Design review of the part built by this model. Coordinates are the model's own, in mm. Face numbers are marked on the shaded views. A direction names the side the tool comes from. Give positions to 0.01 mm unless a question says otherwise; leave off trailing zeros. Loops run counter-clockwise (first coordinate to the right, second up) from the corner with the lowest first, then second, coordinate; pieces in that order, holes last.
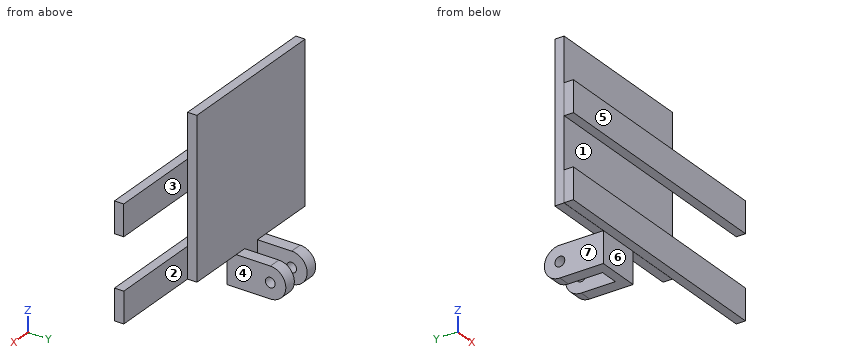
from build123d import *

# Parameters (mm, degrees)
SKETCH1_W           = 6
SKETCH1_H           = 10.023203152
BOSS_EXTRUDE1_DEPTH = 3
SKETCH1_3_W         = 4
SKETCH1_3_H         = 10.023203152
BOSS_EXTRUDE2_DEPTH = 19.05
SKETCH2_R           = 1.5875
CUT_EXTRUDE1_DEPTH  = 19.05
SKETCH3_W           = 80.796379589
SKETCH3_H           = 10
BOSS_EXTRUDE3_DEPTH = 3


with BuildPart() as part:
    # Sketch1 → Boss-Extrude1 (new body)
    with BuildSketch(Plane(origin=(0, 0, 0), x_dir=(1, 0, 0), z_dir=(0, 1, 0))):
        Polygon((0, 50.8), (0, 0), (50.8, 0), (50.8, 50.8), (32.4, 50.8), (28.4, 50.8), (22.4, 50.8), (18.4, 50.8), align=None)
        with Locations((25.4, 55.811601576)):
            Rectangle(SKETCH1_W, SKETCH1_H)
    extrude(amount=BOSS_EXTRUDE1_DEPTH)

    # Sketch1_3 → Boss-Extrude2 (add)
    with BuildSketch(Plane(origin=(0, 0, 0), x_dir=(1, 0, 0), z_dir=(0, 1, 0))):
        with Locations((30.4, 55.811601576)):
            Rectangle(SKETCH1_3_W, SKETCH1_3_H)
        with Locations((20.4, 55.811601576)):
            Rectangle(SKETCH1_3_W, SKETCH1_3_H)
    extrude(amount=BOSS_EXTRUDE2_DEPTH)

    # Sketch2 → Cut-Extrude1 (cut)
    with BuildSketch(Plane(origin=(32.4, 0, 0), x_dir=(0, 0, -1), z_dir=(1, 0, 0))):
        with Locations((55.811601576, 14.038398424)):
            Circle(SKETCH2_R)
        with BuildLine():
            Line((50.8, 14.038398424), (49.911458456, 20.395059664))
            Line((49.911458456, 20.395059664), (64.501767063, 21.247740037))
            Line((64.501767063, 21.247740037), (60.823203152, 14.038398424))
            ThreePointArc((60.823203152, 14.038398424), (55.811601576, 19.05), (50.8, 14.038398424))
        make_face()
    extrude(amount=-CUT_EXTRUDE1_DEPTH, mode=Mode.SUBTRACT)

    # Sketch3 → Boss-Extrude3 (add)
    with BuildSketch(Plane.XZ):
        Polygon((30.017240132, -14.222777316), (0.017240132, -14.222777316), (0.017240132, -24.222777316), (80.817240132, -24.222777316), (80.817240132, -14.222777316), align=None)
        with Locations((40.354723884, -45.757439596)):
            Rectangle(SKETCH3_W, SKETCH3_H)
    extrude(amount=BOSS_EXTRUDE3_DEPTH)


solid = part.part
Q1. Take a section at B-B (x = 31). Give the boundary of the cut face in (y, z) (1 decimal).
Results:
outline: (-3, -50.8) - (0, -50.8) - (0, -60.8) - (14, -60.8) arc R5 ccw to (14, -50.8) - (3, -50.8) - (3, 0) - (0, 0) - (0, -14.2) - (-3, -14.2) - (-3, -24.2) - (0, -24.2) - (0, -40.8) - (-3, -40.8) - close; hole circle Ø3.2 at (14, -55.8)
Q2. Draft analysis for pull direction Z (two halves, no side actions). For the marked faces 1 and 2, state which applies: pulls with the +Z half, pulls with the -Z half, needs draft (parallel to the pull), parting line crosses it, or undercut.
Results:
face 1: undercut
face 2: needs draft
Q3. Take a section at D-D (y = 7.75). Give the boundary of the cut face in (x, z), plus the area to 3 significant figures.
Results:
outline: (18.4, -60.82) - (22.4, -60.82) - (22.4, -50.8) - (18.4, -50.8) - close; (28.4, -60.82) - (32.4, -60.82) - (32.4, -50.8) - (28.4, -50.8) - close
area: 80.2 mm2
Q4. Take a section at A-A (x = 73). Give the boundary of the cut face in (y, z).
Results:
outline: (-3, -50.76) - (0, -50.76) - (0, -40.76) - (-3, -40.76) - close; (-3, -24.22) - (0, -24.22) - (0, -14.22) - (-3, -14.22) - close
Q5. Insertion check: pin 1 (6 mm diameter, centred on x = 46, z = -45.5, fed in from +Y); pin 2 (11 mm diameter, centred on y = 13.5, z = -54, fed in from -X); pin 3 (0.9 mm diameter, centred on y = -1, z = -45, fed in from +X). Each pin has a flat end and moves straight along its axis. Give the tip position at first contact, or say it passes through.
Results:
pin 1: stops at y = 3
pin 2: stops at x = 18.4
pin 3: stops at x = 80.75
Q6. Tool access review of the marked faces 3, 4, 5, 6 and 7: name each direction out of +Z, -Z, +X, -X, +Y, -Y from which nothing blocks a thin tool from reaching the whole face with its end or side.
Results:
face 3: +Z, -Z, +X, +Y
face 4: -Z, +X, +Y, -Y
face 5: +Z, -Z, +X, -X, -Y
face 6: -Z, +X, -X, -Y
face 7: -Z, -X, +Y, -Y
Q7. Wall thickness on line 1 (Y direction, x = 5.5, z = -47); line 2 (Y direction, x = 9.5, z = -30.5); line 3 (X direction, y = 2, z = -17): over which ranges is each line inside the solid? List them lowest first.
Results:
line 1: y = -3 to 3
line 2: y = 0 to 3
line 3: x = 0 to 50.8
